from build123d import *

# Parameters (mm, degrees)
F1_DEPTH = 127
F3_DEPTH = 32.67148


with BuildPart() as f1:
    # F0 (on Right) → F1 (new body)
    with BuildSketch(Plane.YZ):
        Polygon((-3.369482, -22.250649), (-3.369482, 41.249351), (-41.469482, -22.250649), align=None)
    extrude(amount=-F1_DEPTH)

    # F2 (on face) → F3 (cut, through all)
    with BuildSketch(Plane(origin=(0, -20.675804, 12.405482), x_dir=(1, 0, 0), z_dir=(0, -0.857493, 0.514496))):
        Polygon((-127, -40.415646), (0, -40.415646), (-63.5, -3.753904), align=None)
    extrude(amount=-F3_DEPTH, mode=Mode.SUBTRACT)


solid = f1.part
The listing builds one solid part. Answer for the finished solid, in the listing's coordinates (mm). Coordinates: 2 decimals unless noted, no trailing zeros. Loops run counter-clockwise (first coordinate to the right, second up) from the corner with the lowest first, then second, coordinate; pieces in that order, holes last. Notation, with made-up numbers: M 72.25,79.5 L 115.25,79.5 A18 ccw 115.25,112.5 Z; hole C -37,42.25 d9. An arc over 180 degrees is marked long. Answer in a Markdown table with one row per item.
1) Find section C-C (y = -9.5). Determine the outline of the cut face in (x, z), then the cut area to 3 significant figures.
Answers below:
| item | result |
|---|---|
| outline | M -127,-22.25 L -98.51,-22.25 L -63.5,1.32 L -28.49,-22.25 L 0,-22.25 L 0,31.03 L -127,31.03 Z |
| area | 5,940 mm^2 |
2) Find section B-B (y = -30). Determine the outline of the cut face in (x, z).
Answers below:
| item | result |
|---|---|
| outline | M -127,-22.25 L -116.78,-22.25 L -88.39,-3.13 L -127,-3.13 Z; M -38.61,-3.13 L -10.22,-22.25 L 0,-22.25 L 0,-3.13 Z |
3) Find the intervals of material crossed by probe 1 along X at (y, z) = (-13, -19); probe 2 along X at (y, z) = (-22.5, -17); probe 3 along Y at (x, z) = (-84, 16.5), in increasing order.
Answers below:
| item | result |
|---|---|
| probe 1 | -127 to -96.8, -30.2 to 0 |
| probe 2 | -127 to -102.3, -24.7 to 0 |
| probe 3 | -18.22 to -3.37 |
4) Given pin 1 (4 mm diameter, centred on x = -83, y = -8.5, fed in from +Z); pin 2 (3 mm diameter, centred on x = -89.5, z = 34.5, fed in from -Y); pin 3 (1 mm diameter, centred on x = -38.5, z = 4.5, fed in from -Y), each flat-ended and moving along its own axis, determine where each tip first touches the part or whether it passes through.
Answers below:
| item | result |
|---|---|
| pin 1 | z = 36.03 |
| pin 2 | y = -8.32 |
| pin 3 | y = -25.72 |
5) Find section D-D (x = -118.5). Determine the outline of the cut face in (y, z).
Answers below:
| item | result |
|---|---|
| outline | M -38.94,-18.04 L -31.93,-22.25 L -3.37,-22.25 L -3.37,41.25 Z |
6) Find section A-A (z = -12.5). Determine the outline of the cut face in (x, y).
Answers below:
| item | result |
|---|---|
| outline | M -127,-35.62 L -107.3,-35.62 L -78.57,-3.37 L -127,-3.37 Z; M -48.43,-3.37 L -19.7,-35.62 L 0,-35.62 L 0,-3.37 Z |
7) Determine the mould class of faces 1 (the flat face through (-38.361, -19.376, -9.678)), 2 (the flat face through (0, -14, -4)), 3 (the flat face through (-87.75, -19.11, -9.24)), 4 (the flat face through (-62.61, -17.92, 17)) for opening direction X: released by +X, released by -X, zero draft, split by the parting line, or undercut.
Answers below:
| item | result |
|---|---|
| face 1 | undercut |
| face 2 | released by +X |
| face 3 | undercut |
| face 4 | zero draft |
